```python
from build123d import *

# Parameters (mm, degrees)
F0_W      = 203.2
F0_H      = 457.2
F1_DEPTH  = 19.05
F2_R      = 19.04999
F3_R      = 19.04999
F5_DEPTH  = 5
F6_R      = 73.5
F7_DEPTH  = 25.4
F8_SIZE   = 6.35
F9_R      = 36
F10_DEPTH = 3
F11_R     = 29
F12_DEPTH = 25.4
F13_R     = 53.975
F14_DEPTH = 25.4


# Not quite as in the source:
# - a fillet or chamfer is up to 0.001 mm smaller than in the source, because OpenCascade refuses the exact size


with BuildPart() as f1:
    # F0 (on Front) → F1 (new body)
    with BuildSketch(Plane.XZ):
        Rectangle(F0_W, F0_H)
    extrude(amount=F1_DEPTH)

    # F2 (radius 19.05 in the source; OpenCascade refuses exactly that, so slightly less here)
    f2_edges = [f1.edges().sort_by_distance(p)[0] for p in [
        (-101.6, -19.05, 0),
    ]]
    fillet(f2_edges, radius=F2_R)

    # F3 (radius 19.05 in the source; OpenCascade refuses exactly that, so slightly less here)
    f3_edges = [f1.edges().sort_by_distance(p)[0] for p in [
        (101.6, -19.05, 0),
    ]]
    fillet(f3_edges, radius=F3_R)

    # F4 (on face) → F5 (cut)
    with BuildSketch(Plane.XZ.offset(19.05)):
        with BuildLine():
            Line((82, 3.0169707144), (82, 47.7830292856))
            ThreePointArc((82, 47.7830292856), (0, 110.4), (-82, 47.7830292856))
            Line((-82, 47.7830292856), (-82, 3.0169707144))
            ThreePointArc((-82, 3.0169707144), (0, -59.6), (82, 3.0169707144))
        make_face()
    extrude(amount=-F5_DEPTH, mode=Mode.SUBTRACT)

    # F6 (on face) → F7 (cut)
    with BuildSketch(Plane.XZ.offset(19.05)):
        with Locations((0, 25.4)):
            Circle(F6_R)
    extrude(amount=-F7_DEPTH, mode=Mode.SUBTRACT)

    # F8
    f8_edges = [f1.edges().sort_by_distance(p)[0] for p in [
        (-73.5, 0, 25.4),
    ]]
    chamfer(f8_edges, length=F8_SIZE)

    # F9 (on face) → F10 (cut)
    with BuildSketch(Plane.XZ.offset(19.05)):
        with Locations((0, 150.4)):
            Circle(F9_R)
    extrude(amount=-F10_DEPTH, mode=Mode.SUBTRACT)

    # F11 (on face) → F12 (cut)
    with BuildSketch(Plane.XZ.offset(19.05)):
        with Locations((0, 150.4)):
            Circle(F11_R)
    extrude(amount=-F12_DEPTH, mode=Mode.SUBTRACT)

    # F13 (on face) → F14 (cut)
    with BuildSketch(Plane.XZ.offset(19.05)):
        with Locations((0, -155.575)):
            Circle(F13_R)
    extrude(amount=-F14_DEPTH, mode=Mode.SUBTRACT)


solid = f1.part
```
Here's how the part is built. I have some questions about the finished solid (model axes, mm). A direction names the side the tool comes from. Coordinates: 2 decimals unless noted, no trailing zeros. Loops run counter-clockwise (first coordinate to the right, second up) from the corner with the lowest first, then second, coordinate; pieces in that order, holes last. Notation, with made-up numbers: (52.5, 81.25) - (83.5, 81.25) arc R18 cw to (83.5, 94.25) - close; hole circle Ø2 at (76.5, 16). An arc over 180 degrees is marked (long way). Return JSON: item names as keys, results as strings. Group by question number.
Item 1: Will these pins go through, and if not, where does the flat tip stop? P1, Ø4, axis at x = 56, z = -142, coming from the +Y side; P2, Ø5.5, axis at y = -17.5, z = 25, coming from the -X side; P3, Ø21.5, axis at x = 7.5, z = 139.5, coming from the -Y side; P4, Ø2.5, axis at y = -16.5, z = 29.5, coming from the +X side.
Item 2: On a 3-axis mill with a long thin cutter (end or side, diameter ignored), from which of +Z, -Z, +X, -X, +Y, -Y can I reach the whole of each face in a straight line? I mean faces 4 (the face through (-56, -19.05, -48)), 5 (the face through (-24, -16.05, 167)). Say none if no direction works.
Item 3: We'd pull the mould along Z, two halves only. Please class faces 1 (the face through (95.87, -13.62, 3.2)), 2 (the face through (-11.701, -9.658, -208.266)), 3 (the face through (-1, -9, 228.6)): +Z half, -Z half, draft (parallel to the pull), parting line (faces both ways), or undercut.
Item 4: I need wall thicknesses on line 1 (Z direction, x = 0, y = -17); line 2 (Z direction, x = 1, y = -15); line 3 (Z direction, x = 44.5, y = -11.25). Which ranges of each line are inside material? Lowest first, please. Write a range as from..to.
Item 5: If we section it at C-C on x = -47: State how many separate pieces and enclosed holes the cut face has, and give its area (3 significant figures).
Item 6: If we section it at B-B on x = 0: Write out the boundary of the cut face in (y, z).
Calculated:
{
 "1": {"P1": "stops at y = 0", "P2": "stops at x = -94.61", "P3": "passes through", "P4": "stops at x = 93.97"},
 "2": {"face 4": "+Z, -Z, +X, -X, -Y", "face 5": "-Y"},
 "3": {"face 1": "draft", "face 2": "undercut", "face 3": "+Z half"},
 "4": {"line 1": "z = -228.6..-209.55, -101.6..-59.6, 110.4..114.4, 186.4..228.6", "line 2": "z = -228.6..-209.54, -101.61..-59.59, 110.39..121.42, 179.38..228.6", "line 3": "z = -228.6..-186.12, -125.03..-33.1, 83.9..228.6"},
 "5": {"separate pieces": "3", "enclosed holes": "0", "area": "5,350 mm^2"},
 "6": {"outline": "(-19.05, -228.6) - (0, -228.6) - (0, -209.55) - (-19.05, -209.55) - close; (-19.05, -101.6) - (0, -101.6) - (0, -54.45) - (-6.35, -48.1) - (-14.05, -48.1) - (-14.05, -59.6) - (-19.05, -59.6) - close; (-19.05, 110.4) - (-14.05, 110.4) - (-14.05, 98.9) - (-6.35, 98.9) - (0, 105.25) - (0, 121.4) - (-16.05, 121.4) - (-16.05, 114.4) - (-19.05, 114.4) - close; (-19.05, 186.4) - (-16.05, 186.4) - (-16.05, 179.4) - (0, 179.4) - (0, 228.6) - (-19.05, 228.6) - close"}
}
